Part model, mm, in its own coordinate system. Give positions to 0.01 mm unless a question says otherwise; leave off trailing zeros. Write each loop counter-clockwise with the first axis right and the second up, starting at its lowest first coordinate (ties: lowest second). Pieces come first, ordered by that corner, then holes. Notation, with made-up numbers: (16.25, -16.75) - (47.25, -16.75) arc R17 cw to (47.25, -11.75) - close; hole circle Ø10 at (13.25, 47.25). An arc over 180 degrees is marked (long way). Answer in a Markdown table with one row per item. Add a question column.
1. Band-saw the part on B-B on z = -31.5. Write the cut outline in (x, y).
2. Probe line 1 along X through (y, z) = (-2.3, -20.5); line 2 along X through (y, z) = (-4.4, 0.5); line 3 along Z through (x, y) = (14.5, -3.55). List the from-to ranges inside material, lowest first.
3. Band-saw the part on A-A on y = -1.3. Write the cut outline in (x, z), plus the area to 3 significant figures.
4. Drop flat-ended pins along their axis: pin 1 Ø1.5 at (x, y) = (-3.5, -3.5) entering from +Z; pin 2 Ø2 at (x, y) = (-9, -1.5) entering from +Z; pin 3 Ø1.5 at (y, z) = (-2.5, -26) entering from -X. Give the stop position or say it passes through.
5. Band-saw the part on C-C on x = 14. Write the cut outline in (y, z).
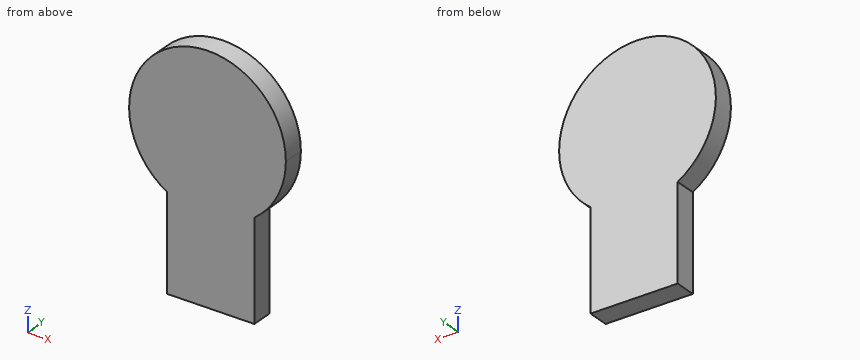
```python
from build123d import *

# Parameters (mm, degrees)
F1_DEPTH = 5


with BuildPart() as f1:
    # F0 (on Front) → F1 (new body)
    with BuildSketch(Plane.XZ):
        with BuildLine():
            ThreePointArc((11.016843, -14.734487), (0.947342, -18.373309), (-9.443007, -15.789413))
            Line((-9.443007, -15.789413), (-9.443007, -38.137238))
            Line((-9.443007, -38.137238), (11.016843, -38.137238))
            Line((11.016843, -38.137238), (11.016843, -14.734487))
        make_face()
        with BuildLine():
            Line((-9.443007, 0), (-9.443007, -15.789413))
            ThreePointArc((-9.443007, -15.789413), (0.947342, -18.373309), (11.016843, -14.734487))
            Line((11.016843, -14.734487), (11.016843, 0))
            Line((11.016843, 0), (-9.443007, 0))
        make_face()
        with BuildLine():
            ThreePointArc((11.016843, -14.734487), (16.449327, -8.239879), (18.397716, 0))
            ThreePointArc((18.397716, 0), (-9.075962, 16.003214), (-9.443007, -15.789413))
            Line((-9.443007, -15.789413), (-9.443007, 0))
            Line((-9.443007, 0), (11.016843, 0))
            Line((11.016843, 0), (11.016843, -14.734487))
        make_face()
    extrude(amount=F1_DEPTH)


solid = f1.part
```
Values:
| question | item | result |
|---|---|---|
| 1 | outline | (-9.44, -5) - (11.02, -5) - (11.02, 0) - (-9.44, 0) - close |
| 2 | line 1 | x = -9.44 to 11.02 |
| 2 | line 2 | x = -18.39 to 18.39 |
| 2 | line 3 | z = -11.32 to 11.32 |
| 3 | outline | (-9.44, -38.14) - (11.02, -38.14) - (11.02, -14.73) arc R18.4 ccw to (18.4, 0) arc R18.4 ccw (long way) to (-9.44, -15.79) - close |
| 3 | area | 1,490 mm² |
| 4 | pin 1 | stops at z = 18.19 |
| 4 | pin 2 | stops at z = 16.57 |
| 4 | pin 3 | stops at x = -9.44 |
| 5 | outline | (-5, -11.94) - (0, -11.94) - (0, 11.94) - (-5, 11.94) - close |
